Work out the finished part from the listing and answer in its coordinate system (mm). Coordinates: 2 decimals unless noted, no trailing zeros. Loops run counter-clockwise (first coordinate to the right, second up) from the corner with the lowest first, then second, coordinate; pieces in that order, holes last. Notation, with made-up numbers: (8.25, 36.5) -> (37.25, 36.5) arc R13 cw to (37.25, 50.5) -> close; hole circle Ø10 at (85.5, 48.25). An arc over 180 degrees is marked (long way). One line per question, with ' | ' between items.
Autodesk Inventor part; units mm, degrees
ref_plane "YZ Plane" through (0, 0, 0) normal (1, 0, 0) x (0, 1, 0)
ref_plane "XZ Plane" through (0, 0, 0) normal (0, 1, 0) x (-1, 0, 0)
ref_plane "XY Plane" through (0, 0, 0) normal (0, 0, 1) x (1, 0, 0)
sketch "Эскиз2" plane through (0, 0, 0) normal (0, 1, 0) x (-1, 0, 0)
  line L0 (3, 5) -> (-3, 5)
  line L1 (-3, 5) -> (-3, -5)
  line L2 (-3, -5) -> (3, -5)
  line L3 (3, -5) -> (3, 5)
  line L4 (3, 0) -> (-3, 0) construction
  line L5 (0, 5) -> (0, -5) construction
  circle A0 centre (0, 0) radius 1.25
  dimension "d0" = 6
  dimension "d1" = 10
  dimension "d2" = 2.5
extrude "Выдавливание1" add sketch "Эскиз2" along normal blind 10 contours L3 L2 L1 L0 | A0
sketch "Эскиз4" plane through (-3, 0, 5) normal (0, 0, 1) x (1, 0, 0)
  line L0 (3, 0) -> (3, 10) construction
  line L1 (6, 10) -> (0, 10) construction
  line L2 (0, 0) -> (0, 10) construction
  line L3 (0, 5) -> (6, 5) construction
  line L4 (6, 0) -> (6, 10) construction
  circle A0 centre (3, 5) radius 1.25
  dimension "d8" = 2.5
extrude "Выдавливание3" cut sketch "Эскиз4" against normal blind 10
fillet "Сопряжение1" radius 0.5 4 edges at (-3, 10, 0) (0, 10, 5) (3, 10, 0) (0, 10, -5)
properties part number "pusher"
1) The mould has two halves that part along Y. Classify faces 1 (the face through (0, 10, 0)), 2 (the face through (0, 0, 0)), 3 (the face through (-0.27, 3.78, 0.07)), 4 (the face through (-1, 4, -5)): released by +Y, released by -Y, zero draft, split by the parting line, or undercut.
Check values:
face 1: released by +Y | face 2: released by -Y | face 3: undercut | face 4: zero draft
2) Find section B-B (y = 5). Write down the section's boundary in (x, z), plus the area to 3 significant figures.
Check values:
outline: (-3, -5) -> (-1.25, -5) -> (-1.25, 5) -> (-3, 5) -> close; (1.25, -5) -> (3, -5) -> (3, 5) -> (1.25, 5) -> close | area: 35.0 mm^2
3) Find the intervals of material crossed by line 1 along Y through (x, z) = (0, -1.5); line 2 along Y through (x, z) = (-0.5, 1.75); line 3 along X through (y, z) = (4.5, 1), in increasing order.
Check values:
line 1: y = 0 to 3.75, 6.25 to 10 | line 2: y = 0 to 3.85, 6.15 to 10 | line 3: x = -3 to -1.15, 1.15 to 3
4) A flat-ended cylindrical pin translates along its axis: pin 1 (1 mm diameter, centred on x = -0.5, y = 5, fed in from +Z). Find the tip coordinate at first contact, or state that the pin passes through.
Check values:
pin 1: passes through
5) Find section A-A (x = 0.75). Write down the section's boundary in (y, z).
Check values:
outline: (0, -5) -> (4, -5) -> (4, 5) -> (0, 5) -> close; (6, -5) -> (9.5, -5) arc R0.5 ccw to (10, -4.5) -> (10, 4.5) arc R0.5 ccw to (9.5, 5) -> (6, 5) -> close
6) Find section D-D (x = 0). Write down the section's boundary in (y, z), plus the area to 3 significant figures.
Check values:
outline: (0, -5) -> (3.75, -5) -> (3.75, 5) -> (0, 5) -> close; (6.25, -5) -> (9.5, -5) arc R0.5 ccw to (10, -4.5) -> (10, 4.5) arc R0.5 ccw to (9.5, 5) -> (6.25, 5) -> close | area: 74.9 mm^2
7) Find section C-C (z = 2.5). Write down the section's boundary in (x, y).
Check values:
outline: (-3, 0) -> (3, 0) -> (3, 9.5) arc R0.5 ccw to (2.5, 10) -> (-2.5, 10) arc R0.5 ccw to (-3, 9.5) -> close; hole circle Ø2.5 at (0, 5)
